Source: three-view drawing plus pictorial views. Frame: mm from the lowest corner of the part. Give positions to 0.01 mm unless a question says otherwise; leave off trailing zeros. Write each loop counter-clockwise with the first axis right and the second up, starting at its lowest first coordinate (ties: lowest second). Pieces come first, ordered by that corner, then holes.
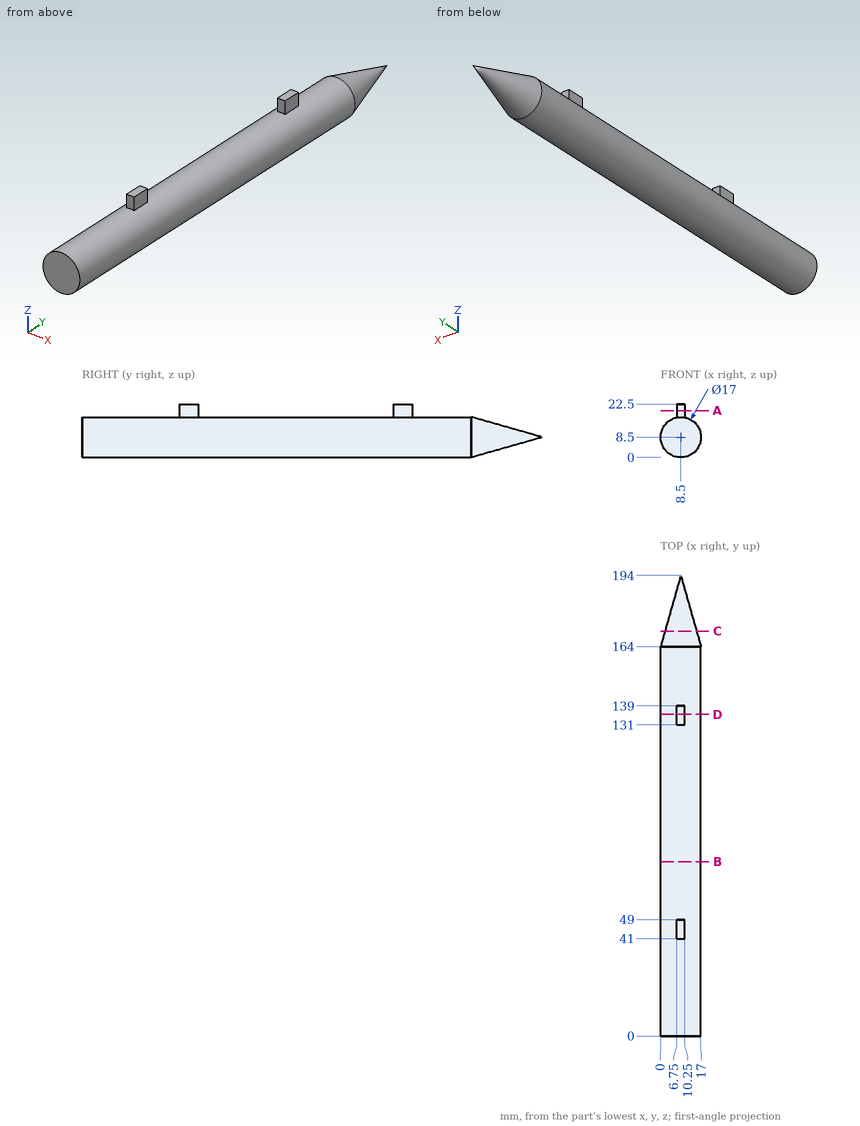
Q1. Ray query, line 1 along Y through (x, z) = (7, 21.5); line 2 along Z through (x, y) = (8, 54); line 3 along X through (y, z) = (123, 6.5). Return the intervals inside material, ascending.
Filled sheet:
line 1: y = 41 to 49, 131 to 139
line 2: z = 0.01 to 16.99
line 3: x = 0.24 to 16.76
Q2. Pin query (flat end, axial travel): P1, Ø1.7, axis at y = 135, z = 20, coming from the -X side; P2, Ø3, axis at x = 8.5, z = 20, coming from the +Y side; P3, Ø4, axis at x = 8, z = 19.5, coming from the -Y side; P4, Ø6, axis at x = 2, z = 19, coming from the +Y side. Return the tip coordinate at first contact, or that it passes through.
Filled sheet:
P1: stops at x = 6.75
P2: stops at y = 139
P3: stops at y = 41
P4: passes through
Q3. Section D-D on y = 135.5. Output: boundary loops of the cut face in (x, z), plus the area to 3 significant figures.
Filled sheet:
outline: (6.75, 16.82) arc R8.5 ccw (long way) to (10.25, 16.82) - (10.25, 22.5) - (6.75, 22.5) - close
area: 246 mm2
Q4. Section A-A on z = 19.75. Output: boundary loops of the cut face in (x, y), plus the area to 3 significant figures.
Filled sheet:
outline: (6.75, 41) - (10.25, 41) - (10.25, 49) - (6.75, 49) - close; (6.75, 131) - (10.25, 131) - (10.25, 139) - (6.75, 139) - close
area: 56.0 mm2
Q5. Section B-B on y = 73.5. Output: boundary loops of the cut face in (x, z), plus the area to 3 significant figures.
Filled sheet:
outline: circle Ø17 at (8.5, 8.5)
area: 227 mm2
Q6. Section C-C on y = 170.5. Output: boundary loops of the cut face in (x, z), plus the area to 3 significant figures.
Filled sheet:
outline: circle Ø13.32 at (8.5, 8.5)
area: 139 mm2
